from build123d import *

# Parameters (mm, degrees)
SKETCH_1_W          = 30
SKETCH_1_H          = 48
EXTRUDE_1_DEPTH     = 7
FILLET_1_R          = 2
FILLET_2_R          = 2
SKETCH_2_W          = 26
SKETCH_2_H          = 3
CUT_EXTRUDE_1_DEPTH = 4


with BuildPart() as part:
    # Эскиз1 → Бобышка-Вытянуть1 (new body)
    with BuildSketch(Plane(origin=(0, 0, 0), x_dir=(1, 0, 0), z_dir=(0, 1, 0))):
        Rectangle(SKETCH_1_W, SKETCH_1_H)
    extrude(amount=EXTRUDE_1_DEPTH)

    # Скругление1
    fillet_1_edges = [part.edges().sort_by_distance(p)[0] for p in [
        (-15, 7, 0),
        (0, 7, 24),
        (15, 7, 0),
        (0, 0, 24),
        (-15, 0, 0),
        (0, 0, -24),
        (15, 0, 0),
        (0, 7, -24),
    ]]
    fillet(fillet_1_edges, radius=FILLET_1_R)

    # Скругление2
    # the kernel refuses this fillet: 2 mm, written as the material it takes off along each edge
    with BuildSketch(Plane(origin=(13, 2, 22), x_dir=(1, 0, 0), z_dir=(0, 0, 1))) as fillet_2_piece_1_section:
        Polygon((0, 0), (FILLET_2_R, 0), (FILLET_2_R, -FILLET_2_R), (0, -FILLET_2_R), align=None)
    fillet_2_piece_1 = extrude(amount=FILLET_2_R, mode=Mode.PRIVATE)
    fillet_2_piece_1 = fillet_2_piece_1 - Plane(origin=(13, 2, 22), x_dir=(-0.7071067811865475, 0.7071067811865475, 0), z_dir=(0, 0, 1)) * Sphere(FILLET_2_R, mode=Mode.PRIVATE)
    add(fillet_2_piece_1, mode=Mode.SUBTRACT)
    with BuildSketch(Plane(origin=(-13, 2, 22), x_dir=(-1, 0, 0), z_dir=(0, 0, 1))) as fillet_2_piece_2_section:
        Polygon((0, 0), (FILLET_2_R, 0), (FILLET_2_R, FILLET_2_R), (0, FILLET_2_R), align=None)
    fillet_2_piece_2 = extrude(amount=FILLET_2_R, mode=Mode.PRIVATE)
    fillet_2_piece_2 = fillet_2_piece_2 - Plane(origin=(-13, 2, 22), x_dir=(0.7071067811865475, 0.7071067811865475, 0), z_dir=(0, 0, 1)) * Sphere(FILLET_2_R, mode=Mode.PRIVATE)
    add(fillet_2_piece_2, mode=Mode.SUBTRACT)
    with BuildSketch(Plane(origin=(13, 2, -22), x_dir=(0, 0, -1), z_dir=(1, 0, 0))) as fillet_2_piece_3_section:
        Polygon((0, 0), (FILLET_2_R, 0), (FILLET_2_R, -FILLET_2_R), (0, -FILLET_2_R), align=None)
    fillet_2_piece_3 = extrude(amount=FILLET_2_R, mode=Mode.PRIVATE)
    fillet_2_piece_3 = fillet_2_piece_3 - Plane(origin=(13, 2, -22), x_dir=(0, 0.7071067811865475, 0.7071067811865475), z_dir=(1, 0, 0)) * Sphere(FILLET_2_R, mode=Mode.PRIVATE)
    add(fillet_2_piece_3, mode=Mode.SUBTRACT)
    with BuildSketch(Plane(origin=(-13, 2, -22), x_dir=(0, 0, -1), z_dir=(-1, 0, 0))) as fillet_2_piece_4_section:
        Polygon((0, 0), (FILLET_2_R, 0), (FILLET_2_R, FILLET_2_R), (0, FILLET_2_R), align=None)
    fillet_2_piece_4 = extrude(amount=FILLET_2_R, mode=Mode.PRIVATE)
    fillet_2_piece_4 = fillet_2_piece_4 - Plane(origin=(-13, 2, -22), x_dir=(0, 0.7071067811865475, 0.7071067811865475), z_dir=(-1, 0, 0)) * Sphere(FILLET_2_R, mode=Mode.PRIVATE)
    add(fillet_2_piece_4, mode=Mode.SUBTRACT)
    with BuildSketch(Plane(origin=(-13, 5, -22), x_dir=(0, 0, -1), z_dir=(-1, 0, 0))) as fillet_2_piece_5_section:
        Polygon((0, 0), (FILLET_2_R, 0), (FILLET_2_R, -FILLET_2_R), (0, -FILLET_2_R), align=None)
    fillet_2_piece_5 = extrude(amount=FILLET_2_R, mode=Mode.PRIVATE)
    fillet_2_piece_5 = fillet_2_piece_5 - Plane(origin=(-13, 5, -22), x_dir=(0, -0.7071067811865475, 0.7071067811865475), z_dir=(-1, 0, 0)) * Sphere(FILLET_2_R, mode=Mode.PRIVATE)
    add(fillet_2_piece_5, mode=Mode.SUBTRACT)
    with BuildSketch(Plane(origin=(13, 5, -22), x_dir=(0, 0, -1), z_dir=(1, 0, 0))) as fillet_2_piece_6_section:
        Polygon((0, 0), (FILLET_2_R, 0), (FILLET_2_R, FILLET_2_R), (0, FILLET_2_R), align=None)
    fillet_2_piece_6 = extrude(amount=FILLET_2_R, mode=Mode.PRIVATE)
    fillet_2_piece_6 = fillet_2_piece_6 - Plane(origin=(13, 5, -22), x_dir=(0, -0.7071067811865475, 0.7071067811865475), z_dir=(1, 0, 0)) * Sphere(FILLET_2_R, mode=Mode.PRIVATE)
    add(fillet_2_piece_6, mode=Mode.SUBTRACT)
    with BuildSketch(Plane(origin=(-13, 5, 22), x_dir=(-1, 0, 0), z_dir=(0, 0, 1))) as fillet_2_piece_7_section:
        Polygon((0, 0), (FILLET_2_R, 0), (FILLET_2_R, -FILLET_2_R), (0, -FILLET_2_R), align=None)
    fillet_2_piece_7 = extrude(amount=FILLET_2_R, mode=Mode.PRIVATE)
    fillet_2_piece_7 = fillet_2_piece_7 - Plane(origin=(-13, 5, 22), x_dir=(0.7071067811865475, -0.7071067811865475, 0), z_dir=(0, 0, 1)) * Sphere(FILLET_2_R, mode=Mode.PRIVATE)
    add(fillet_2_piece_7, mode=Mode.SUBTRACT)
    with BuildSketch(Plane(origin=(13, 5, 22), x_dir=(1, 0, 0), z_dir=(0, 0, 1))) as fillet_2_piece_8_section:
        Polygon((0, 0), (FILLET_2_R, 0), (FILLET_2_R, FILLET_2_R), (0, FILLET_2_R), align=None)
    fillet_2_piece_8 = extrude(amount=FILLET_2_R, mode=Mode.PRIVATE)
    fillet_2_piece_8 = fillet_2_piece_8 - Plane(origin=(13, 5, 22), x_dir=(-0.7071067811865475, -0.7071067811865475, 0), z_dir=(0, 0, 1)) * Sphere(FILLET_2_R, mode=Mode.PRIVATE)
    add(fillet_2_piece_8, mode=Mode.SUBTRACT)
    with BuildSketch(Plane(origin=(-15, 2, -24), x_dir=(0, 0, 1), z_dir=(0, 1, 0)), Plane(origin=(-15, 2, 24), x_dir=(1, 0, 0), z_dir=(0, 1, 0))) as fillet_2_piece_9:
        with BuildLine():
            CenterArc((FILLET_2_R, FILLET_2_R), FILLET_2_R, 180, 90)
            Line((0, FILLET_2_R), (0, 0))
            Line((0, 0), (FILLET_2_R, 0))
        make_face()
    extrude(amount=3, mode=Mode.SUBTRACT)
    with BuildSketch(Plane(origin=(15, 2, -24), x_dir=(0, 0, 1), z_dir=(0, 1, 0)), Plane(origin=(15, 2, 24), x_dir=(-1, 0, 0), z_dir=(0, 1, 0))) as fillet_2_piece_10:
        with BuildLine():
            CenterArc((FILLET_2_R, -FILLET_2_R), FILLET_2_R, 90, 90)
            Line((0, -FILLET_2_R), (0, 0))
            Line((0, 0), (FILLET_2_R, 0))
        make_face()
    extrude(amount=3, mode=Mode.SUBTRACT)

    # Эскиз2 → Вырез-Вытянуть1 (cut)
    with BuildSketch(Plane(origin=(0, 7, 0), x_dir=(1, 0, 0), z_dir=(0, 1, 0))):
        with Locations((0, 20.5)):
            Rectangle(SKETCH_2_W, SKETCH_2_H)
        Polygon((-13, 24), (-15.574798144, 24), (-15.574798144, 19), (-13, 19), (-13, 22), (13, 22), (13, 19), (18.278986273, 19), (18.278986273, 24), (13, 24), align=None)
    extrude(amount=-CUT_EXTRUDE_1_DEPTH, mode=Mode.SUBTRACT)


solid = part.part
Check sheet for the modelled part. Datum: model origin and axes. Units: mm. A direction names the side the tool comes from. Round coordinates to 2 decimals unless told otherwise and drop trailing zeros. Order: outer loops, then holes, each group sorted by start corner. A loop starts at its lowest first (then second) coordinate and runs counter-clockwise, first axis right, second up.
(1) Cross-section at D-D, the plane y = 5.75. Enter the section's corners in (x, z), and give its area (3 significant figures).
(2) Cross-section at C-C, the plane y = 1.25. Enter the section's corners in (x, z), and give its area (3 significant figures).
(3) Cross-section at B-B, the plane z = 17. Enter the section's corners in (x, y).
(4) Scan lines: probe 1 along Z at (x, y) = (0, 4.5); probe 2 along X at (y, z) = (1.25, 21); probe 3 along Z at (x, y) = (-6, 1.5). Record each from-to range of solid material in increasing order.
(5) Access from +Z, -Z, +X, -X, +Y, -Y to the whole of each face (thin tool, end or side, straight path). Record for faces 1 (the flat face through (0, 3, -22)), 2 (the cylindrical face through (-14.43, 0.6, -0.31)).
(6) Cross-section at A-A, the plane x = -0.5. Enter the section's corners in (y, z), and give its area (3 significant figures).
(7) Go/stop test with flat-tipped pins: P1, Ø2, axis at x = 5, y = 5.5, coming from the -Z side; P2, Ø1.5, axis at x = -5.5, z = -22.5, coming from the +Y side. Record where each tip stops, or that it passes through.
Check sheet entries:
1. outline: (-14.85, -19) - (14.85, -19) - (14.85, 22) arc R1.85 ccw to (13, 23.85) - (-13, 23.85) arc R1.85 ccw to (-14.85, 22) - close
1. area: 1,270 mm2
2. outline: (-14.85, -22) arc R1.85 ccw to (-13, -23.85) - (13, -23.85) arc R1.85 ccw to (14.85, -22) - (14.85, 22) arc R1.85 ccw to (13, 23.85) - (-13, 23.85) arc R1.85 ccw to (-14.85, 22) - close
2. area: 1,410 mm2
3. outline: (-15, 2) arc R2 ccw to (-13, 0) - (13, 0) arc R2 ccw to (15, 2) - (15, 5) arc R2 ccw to (13, 7) - (-13, 7) arc R2 ccw to (-15, 5) - close
4. probe 1: z = -19 to 24
4. probe 2: x = -14.85 to 14.85
4. probe 3: z = -23.94 to 23.94
5. face 1: -Z, +X, -X, +Y
5. face 2: +Z, -Z, -X, -Y
6. outline: (0, -22) arc R2 ccw to (2, -24) - (3, -24) - (3, -19) - (7, -19) - (7, 22) arc R2 ccw to (5, 24) - (2, 24) arc R2 ccw to (0, 22) - close
6. area: 313 mm2
7. P1: stops at z = -19
7. P2: stops at y = 3
